```python
from build123d import *

# Parameters (mm, degrees)
SKETCH1_W           = 50
SKETCH1_H           = 75
SKETCH1_R           = 12.5
BOSS_EXTRUDE1_DEPTH = 3


with BuildPart() as part:
    # Sketch1 → Boss-Extrude1 (new body)
    with BuildSketch(Plane.XY):
        Polygon((-50, 15), (-50, -15), (0, -15), (50, -15), (50, 15), align=None)
        with Locations((-25, -52.5)):
            Rectangle(SKETCH1_W, SKETCH1_H)
        with Locations((-25, -65)):
            Circle(SKETCH1_R, mode=Mode.SUBTRACT)
    extrude(amount=BOSS_EXTRUDE1_DEPTH)


solid = part.part
```
Model file for the job. Use its own axes, mm. A direction names the side the tool comes from. Round coordinates to 2 decimals unless told otherwise and drop trailing zeros. Order: outer loops, then holes, each group sorted by start corner. A loop starts at its lowest first (then second) coordinate and runs counter-clockwise, first axis right, second up. Notation, with made-up numbers: (65, 81) -> (101, 81) arc R17 ccw to (101, 107) -> close; hole circle Ø3 at (6.5, 18.5). An arc over 180 degrees is marked (long way). Use one line per item in the form item = value.
Item 1: Cut at A-A, the plane y = -65. Write the cut outline in (x, z).
Returned:
outline = (-50, 0) -> (-37.5, 0) -> (-37.5, 3) -> (-50, 3) -> close; (-12.5, 0) -> (0, 0) -> (0, 3) -> (-12.5, 3) -> close
Item 2: Tool access for faces 1 (the face through (0, -53, 1)), 2 (the face through (-12, -25, 0)): list every direction of +Z, -Z, +X, -X, +Y, -Y with a clear straight run to the whole face (end or side of a thin tool).
Returned:
face_1 = +Z, -Z, +X, -Y
face_2 = -Z, +X, -X, +Y, -Y
Item 3: Pull direction X, two halves, no side cores. Call faces 3 (the face through (50, 0, 1)), 4 (the face through (25, -15, 1)), 5 (the face through (-34.21, -56.55, 1.48)): released by +X, released by -X, zero draft, split by the parting line, or undercut.
Returned:
face_3 = released by +X
face_4 = zero draft
face_5 = undercut
Item 4: Flat gauge pins, fed straight in: pin 1 Ø0.9 at (x, z) = (29.5, 1.5) entering from -Y; pin 2 Ø22.5 at (x, y) = (-25, -65) entering from +Z. Where does each tip first touch, or does it go through?
Returned:
pin_1 = -15
pin_2 = through
Item 5: Cut at C-C, the plane z = 0.85. Write the cut outline in (x, y), and give its area (3 significant figures).
Returned:
outline = (-50, -90) -> (0, -90) -> (0, -15) -> (50, -15) -> (50, 15) -> (-50, 15) -> close; hole circle Ø25 at (-25, -65)
area = 6,260 mm^2
Item 6: Cut at B-B, the plane x = -25. Write the cut outline in (y, z).
Returned:
outline = (-90, 0) -> (-77.5, 0) -> (-77.5, 3) -> (-90, 3) -> close; (-52.5, 0) -> (15, 0) -> (15, 3) -> (-52.5, 3) -> close
Item 7: Drill centre lines: line 1 (Y direction, x = -25, z = 1.4); line 2 (X direction, y = -15.5, z = 1.4); line 3 (Y direction, x = 45.5, z = 2.05). Where is each one in solid material? Low to high.
Returned:
line_1 = -90 to -77.5, -52.5 to 15
line_2 = -50 to 0
line_3 = -15 to 15
Item 8: Cut at D-D, the plane x = 40.5. Write the cut outline in (y, z), and give its area (3 significant figures).
Returned:
outline = (-15, 0) -> (15, 0) -> (15, 3) -> (-15, 3) -> close
area = 90.0 mm^2
